Check sheet for the modelled part. Datum: model origin and axes. Units: mm. A direction names the side the tool comes from. Coordinates: 2 decimals unless noted, no trailing zeros. Loops run counter-clockwise (first coordinate to the right, second up) from the corner with the lowest first, then second, coordinate; pieces in that order, holes last. Notation, with made-up numbers: M -3,9.25 L 16,9.25 A18 ccw 16,34.25 Z; hole C -10.75,-16 d6. An arc over 180 degrees is marked long. Answer in a Markdown table with one row per item. Add a question column.
Autodesk Inventor part; units mm, degrees
ref_plane "YZ Plane" through (0, 0, 0) normal (1, 0, 0) x (0, 1, 0)
ref_plane "XZ Plane" through (0, 0, 0) normal (0, 1, 0) x (-1, 0, 0)
ref_plane "XY Plane" through (0, 0, 0) normal (0, 0, 1) x (1, 0, 0)
sketch "Sketch1" plane through (0, 0, 0) normal (0, 1, 0) x (-1, 0, 0)
  circle A0 centre (0, 0) radius 1.5875
  dimension "d0" = 3.175
extrude "Extrusion1" add sketch "Sketch1" along normal blind 12.7
thread "Thread1"
chamfer "Chamfer1" distance 0.254 angle 45 1 edges at (1.5875, 0, 0)
sketch "Sketch3" plane through (0, 12.7, 0) normal (0, 1, 0) x (1, 0, 0)
  circle A0 centre (0, 0) radius 0.9525
  dimension "d11" = 1.905
extrude "Extrusion3" add sketch "Sketch3" along normal blind 12.7
properties part number "burner rodx3 part 1" material "Stainless Steel"
Q1. Cross-section at D-D (y = 15.5). Record the cut outline in (x, z) (1 decimal).
Q2. Cross-section at A-A (z = 0). Record the cut outline in (x, y), plus the area to 3 significant figures.
Q3. Cross-section at C-C (y = 11). Record the cut outline in (x, z) (1 decimal), plus the area to 3 significant figures.
Q4. Thickness scan on L1, parallel to Y at x = -1.15, z = 0.6; L2, parallel to X at y = 20, z = 0; L3, parallel to X at y = 3, z = -0.1. Record the ranges inside material, lowest first.
Q5. Cross-section at B-B (x = 0). Record the cut outline in (y, z).
Q6. Access from +Z, -Z, +X, -X, +Y, -Y to the whole of each face (thin tool, end or side, straight path). Record for faces 1 (the face through (0, 25.4, 0)), 2 (the face through (-1, 12.7, -1)).
Answer key:
| question | item | result |
|---|---|---|
| 1 | outline | C 0,0 d1.9 |
| 2 | outline | M -1.59,0.25 L -1.33,0 L 1.33,0 L 1.59,0.25 L 1.59,12.7 L 0.95,12.7 L 0.95,25.4 L -0.95,25.4 L -0.95,12.7 L -1.59,12.7 Z |
| 2 | area | 64.5 mm^2 |
| 3 | outline | C 0,0 d3.2 |
| 3 | area | 7.92 mm^2 |
| 4 | L1 | 0 to 12.7 |
| 4 | L2 | -0.95 to 0.95 |
| 4 | L3 | -1.58 to 1.58 |
| 5 | outline | M 0,-1.33 L 0.25,-1.59 L 12.7,-1.59 L 12.7,-0.95 L 25.4,-0.95 L 25.4,0.95 L 12.7,0.95 L 12.7,1.59 L 0.25,1.59 L 0,1.33 Z |
| 6 | face 1 | +Z, -Z, +X, -X, +Y |
| 6 | face 2 | +Y |
